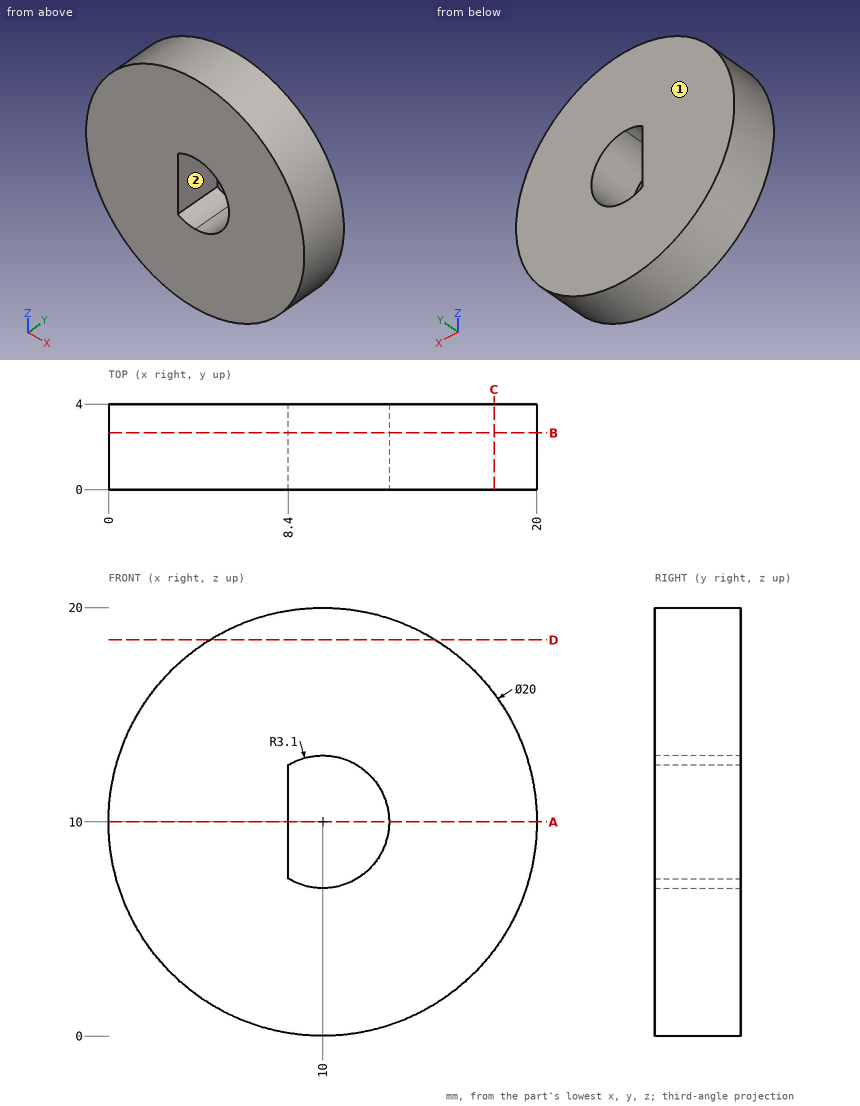
Answer from the drawing. Dimensions are ordinates in mm from the lowest x, y and z of the part. A direction names the side the tool comes from. Round coordinates to 2 decimals unless told otherwise and drop trailing zeros. Write each loop counter-clockwise with the first axis right and the second up, starting at its lowest first coordinate (ties: lowest second). Pieces come first, ordered by that corner, then holes. Notation, with made-up numbers: (86.25, 1.5) -> (142.25, 1.5) arc R34 cw to (142.25, 32.5) -> close; hole circle Ø1 at (5, 33). An arc over 180 degrees is marked (long way). Answer in a Markdown table with one row per item. Add a question column.
1) Which of the six approach directions +Z, -Z, +X, -X, +Y, -Y give full straight-line access (tool end or side, diameter ignored) to the marked faces 1 and 2?
2) Find section D-D, the plane z = 18.5. Determine the outline of the cut face in (x, y).
3) Consider line 1 (X direction, y = 3.45, z = 10); line 2 (X direction, y = 3.45, z = 12); line 3 (Z direction, x = 9.75, y = 0.8). Determine where each line is inside the solid, lowest interval first.
4) Find section A-A, the plane z = 10. Determine the outline of the cut face in (x, y), and give its area (3 significant figures).
5) Find section B-B, the plane y = 2.65. Determine the outline of the cut face in (x, z).
6) Find section C-C, the plane x = 18. Determine the outline of the cut face in (y, z).
7) Given P1, Ø1.2, axis at y = 2, z = 11, coming from the +X side; P2, Ø1.5, axis at x = 7, y = 3, coming from the +Z side; P3, Ø2, axis at y = 3, z = 7, coming from the -X side, each flat-ended and moving along its own axis, determine where each tip first touches the part or whether it passes through.
Findings below:
| question | item | result |
|---|---|---|
| 1 | face 1 | +Z, -Z, +X, -X, +Y |
| 1 | face 2 | +Y, -Y |
| 2 | outline | (4.73, 0) -> (15.27, 0) -> (15.27, 4) -> (4.73, 4) -> close |
| 3 | line 1 | 0 to 8.4, 13.1 to 20 |
| 3 | line 2 | 0.2 to 8.4, 12.37 to 19.8 |
| 3 | line 3 | 0 to 6.91, 13.09 to 20 |
| 4 | outline | (0, 0) -> (8.4, 0) -> (8.4, 4) -> (0, 4) -> close; (13.1, 0) -> (20, 0) -> (20, 4) -> (13.1, 4) -> close |
| 4 | area | 61.2 mm² |
| 5 | outline | circle Ø20 at (10, 10); hole (8.4, 7.34) arc R3.1 ccw (long way) to (8.4, 12.66) -> close |
| 6 | outline | (0, 4) -> (4, 4) -> (4, 16) -> (0, 16) -> close |
| 7 | P1 | x = 19.99 |
| 7 | P2 | z = 19.74 |
| 7 | P3 | x = 0.2 |
